Can you work these out from the model? Positions are in its coordinate system, mm. Face numbers are marked on the shaded views. A direction names the side the tool comes from. Give positions to 0.01 mm unless a question says otherwise; leave off trailing zeros. Order: outer loops, then holes, each group sorted by start corner. A loop starts at its lowest first (then second) coordinate and runs counter-clockwise, first axis right, second up. Notation, with made-up numbers: M -17,1.25 L 30,1.25 A6 cw 30,11.25 Z; hole C 47,21 d4. An arc over 180 degrees is marked long. Use one line per item in the form item = value. Start each with the question number.
1. I need wall thicknesses on L1, parallel to X at y = -2.45, z = -6.35 (3 decimals); L2, parallel to X at y = 29.5, z = 77 (3 decimals); L3, parallel to Z at x = 4, y = 66 (3 decimals). Which ranges of each line are inside material? Lowest first, please.
2. Will these pins go through, and if not, where does the flat tip stop? P1, Ø0.7, axis at y = 1, z = 3, coming from the +X side; P2, Ø7, axis at x = 153, z = 2, coming from the -Y side; P3, Ø1, axis at y = 35, z = 77, coming from the -X side (3 decimals); P4, Ø4, axis at x = 161.925, z = 44.45, coming from the -Y side (3 decimals).
3. I want a section at B-B, the plane z = 27. List the corners of the cut face in (x, y) for me (3 decimals), and give its area (3 significant figures).
4. We'd pull the mould along X, two halves only. Please class the marked faces 1, 2, 3 and 4: +X half, -X half, draft (parallel to the pull), parting line (faces both ways), or undercut.
5. I want a section at D-D, the plane x = 68. List the corners of the cut face in (y, z) for me (3 decimals), and give its area (3 significant figures).
6. I want a section at A-A, the plane z = 50.8. List the corners of the cut face in (x, y) for me (3 decimals), and give its area (3 significant figures).
7. I want a section at C-C, the plane y = 60.5. List the corners of the cut face in (x, z) for me (3 decimals).
8. For the marked faces 5 and 6, which set-ups out of +Z, -Z, +X, -X, +Y, -Y let a thin tool reach every point of the face, with its end or its side?
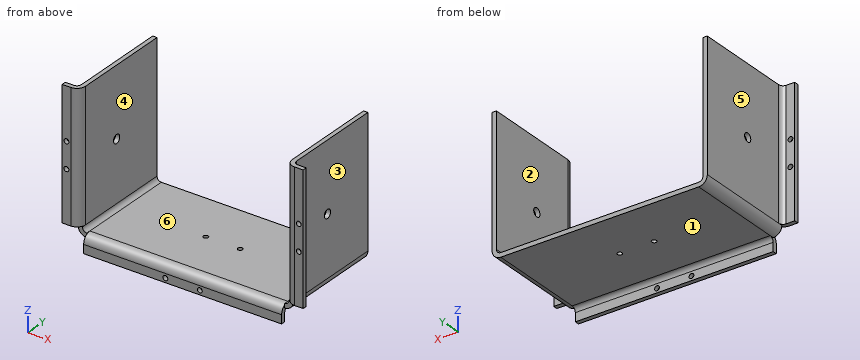
```python
from build123d import *

# Parameters (mm, degrees)
SKETCH1_W                    = 152.4
SKETCH1_H                    = 76.2
BOSS_EXTRUDE1_DEPTH          = 3.175
EDGE_FLANGE5_STRIP_W         = 19.05
EDGE_FLANGE5_STRIP_H         = 3.175
EDGE_FLANGE5_STRIP_CUT_DEPTH = 76.2
EDGE_FLANGE5_DEPTH           = 76.2
EDGE_FLANGE6_STRIP_W         = 19.05
EDGE_FLANGE6_STRIP_H         = 3.175
EDGE_FLANGE6_STRIP_CUT_DEPTH = 76.2
EDGE_FLANGE6_DEPTH           = 76.2
EDGE_FLANGE7_STRIP_W         = 19.05
EDGE_FLANGE7_STRIP_H         = 3.175
EDGE_FLANGE7_STRIP_CUT_DEPTH = 146.05
EDGE_FLANGE7_DEPTH           = 146.05
EDGE_FLANGE8_STRIP_W         = 19.05
EDGE_FLANGE8_STRIP_H         = 3.175
EDGE_FLANGE8_STRIP_CUT_DEPTH = 95.25
EDGE_FLANGE8_DEPTH           = 95.25
EDGE_FLANGE9_STRIP_W         = 19.05
EDGE_FLANGE9_STRIP_H         = 3.175
EDGE_FLANGE9_STRIP_CUT_DEPTH = 95.25
EDGE_FLANGE9_DEPTH           = 95.25
CUT_EXTRUDE1_DEPTH           = 211.820956323
CUT_EXTRUDE1_DEPTH_BACK      = 211.820956323
SKETCH60_R                   = 3.175
CUT_EXTRUDE2_DEPTH           = 207.765399971
CUT_EXTRUDE2_DEPTH_BACK      = 207.765399971
SKETCH61_R                   = 1.778
CUT_EXTRUDE3_DEPTH           = 209.295487229
CUT_EXTRUDE3_DEPTH_BACK      = 209.295487229
SKETCH62_R                   = 1.778


# Sheet-metal steps are written as plain solids
with BuildPart() as part:
    # Sketch1 → Boss-Extrude1 (new body)
    with BuildSketch(Plane.XY):
        with Locations((76.2, 38.1)):
            Rectangle(SKETCH1_W, SKETCH1_H)
    extrude(amount=BOSS_EXTRUDE1_DEPTH)

    # Edge-Flange5 strip (across the edge) → Edge-Flange5 strip cut (cut)
    with BuildSketch(Plane(origin=(152.4, 0, 3.175), x_dir=(-1, 0, 0), z_dir=(0, 1, 0))):
        with Locations((-6.35, -1.5875)):
            Rectangle(EDGE_FLANGE5_STRIP_W, EDGE_FLANGE5_STRIP_H)
    extrude(amount=EDGE_FLANGE5_STRIP_CUT_DEPTH, mode=Mode.SUBTRACT)

    # Edge-Flange5 section (across the edge) → Edge-Flange5 (add)
    with BuildSketch(Plane(origin=(152.4, 0, 3.175), x_dir=(-1, 0, 0), z_dir=(0, 1, 0))):
        with BuildLine():
            Line((-3.175, 3.175), (-3.175, 98.425))
            Line((-3.175, 98.425), (0, 98.425))
            Line((0, 98.425), (0, 3.175))
            ThreePointArc((0, 3.175), (0.92993597, 0.92993597), (3.175, 0))
            Line((3.175, 0), (3.175, -3.175))
            ThreePointArc((3.175, -3.175), (-1.315128061, -1.315128061), (-3.175, 3.175))
        make_face()
    extrude(amount=EDGE_FLANGE5_DEPTH)

    # Edge-Flange6 strip (across the edge) → Edge-Flange6 strip cut (cut)
    with BuildSketch(Plane(origin=(0, 76.2, 3.175), x_dir=(1, 0, 0), z_dir=(0, -1, 0))):
        with Locations((-6.35, -1.5875)):
            Rectangle(EDGE_FLANGE6_STRIP_W, EDGE_FLANGE6_STRIP_H)
    extrude(amount=EDGE_FLANGE6_STRIP_CUT_DEPTH, mode=Mode.SUBTRACT)

    # Edge-Flange6 section (across the edge) → Edge-Flange6 (add)
    with BuildSketch(Plane(origin=(0, 76.2, 3.175), x_dir=(1, 0, 0), z_dir=(0, -1, 0))):
        with BuildLine():
            Line((-3.175, 3.175), (-3.175, 98.425))
            Line((-3.175, 98.425), (0, 98.425))
            Line((0, 98.425), (0, 3.175))
            ThreePointArc((0, 3.175), (0.92993597, 0.92993597), (3.175, 0))
            Line((3.175, 0), (3.175, -3.175))
            ThreePointArc((3.175, -3.175), (-1.315128061, -1.315128061), (-3.175, 3.175))
        make_face()
    extrude(amount=EDGE_FLANGE6_DEPTH)

    # Edge-Flange7 strip (across the edge) → Edge-Flange7 strip cut (cut)
    with BuildSketch(Plane(origin=(149.225, 0, 0), x_dir=(0, 1, 0), z_dir=(-1, 0, 0))):
        with Locations((-6.35, -1.5875)):
            Rectangle(EDGE_FLANGE7_STRIP_W, EDGE_FLANGE7_STRIP_H)
    extrude(amount=EDGE_FLANGE7_STRIP_CUT_DEPTH, mode=Mode.SUBTRACT)

    # Edge-Flange7 section (across the edge) → Edge-Flange7 (add)
    with BuildSketch(Plane(origin=(149.225, 0, 0), x_dir=(0, 1, 0), z_dir=(-1, 0, 0))):
        with BuildLine():
            Line((-3.175, 3.175), (-3.175, 9.525))
            Line((-3.175, 9.525), (0, 9.525))
            Line((0, 9.525), (0, 3.175))
            ThreePointArc((0, 3.175), (0.92993597, 0.92993597), (3.175, 0))
            Line((3.175, 0), (3.175, -3.175))
            ThreePointArc((3.175, -3.175), (-1.315128061, -1.315128061), (-3.175, 3.175))
        make_face()
    extrude(amount=EDGE_FLANGE7_DEPTH)

    # Edge-Flange8 strip (across the edge) → Edge-Flange8 strip cut (cut)
    with BuildSketch(Plane(origin=(155.575, 0, 101.6), x_dir=(0, 1, 0), z_dir=(0, 0, -1))):
        with Locations((-6.35, -1.5875)):
            Rectangle(EDGE_FLANGE8_STRIP_W, EDGE_FLANGE8_STRIP_H)
    extrude(amount=EDGE_FLANGE8_STRIP_CUT_DEPTH, mode=Mode.SUBTRACT)

    # Edge-Flange8 section (across the edge) → Edge-Flange8 (add)
    with BuildSketch(Plane(origin=(155.575, 0, 101.6), x_dir=(0, 1, 0), z_dir=(0, 0, -1))):
        with BuildLine():
            Line((-3.175, 3.175), (-3.175, 9.525))
            Line((-3.175, 9.525), (0, 9.525))
            Line((0, 9.525), (0, 3.175))
            ThreePointArc((0, 3.175), (0.92993597, 0.92993597), (3.175, 0))
            Line((3.175, 0), (3.175, -3.175))
            ThreePointArc((3.175, -3.175), (-1.315128061, -1.315128061), (-3.175, 3.175))
        make_face()
    extrude(amount=EDGE_FLANGE8_DEPTH)

    # Edge-Flange9 strip (across the edge) → Edge-Flange9 strip cut (cut)
    with BuildSketch(Plane(origin=(-3.175, 0, 6.35), x_dir=(0, 1, 0), z_dir=(0, 0, 1))):
        with Locations((-6.35, -1.5875)):
            Rectangle(EDGE_FLANGE9_STRIP_W, EDGE_FLANGE9_STRIP_H)
    extrude(amount=EDGE_FLANGE9_STRIP_CUT_DEPTH, mode=Mode.SUBTRACT)

    # Edge-Flange9 section (across the edge) → Edge-Flange9 (add)
    with BuildSketch(Plane(origin=(-3.175, 0, 6.35), x_dir=(0, 1, 0), z_dir=(0, 0, 1))):
        with BuildLine():
            Line((-3.175, 3.175), (-3.175, 9.525))
            Line((-3.175, 9.525), (0, 9.525))
            Line((0, 9.525), (0, 3.175))
            ThreePointArc((0, 3.175), (0.92993597, 0.92993597), (3.175, 0))
            Line((3.175, 0), (3.175, -3.175))
            ThreePointArc((3.175, -3.175), (-1.315128061, -1.315128061), (-3.175, 3.175))
        make_face()
    extrude(amount=EDGE_FLANGE9_DEPTH)

    # Sketch60 → Cut-Extrude1 (cut, two sides: drawn at the far end of the back side and taken through both)
    with BuildSketch(Plane(origin=(155.575, 0, 0), x_dir=(0, 0, -1), z_dir=(1, 0, 0)).offset(-CUT_EXTRUDE1_DEPTH_BACK)):
        with Locations(Location((-50.8, 34.925, 0), (0, 0, 180))):
            Circle(SKETCH60_R)
    extrude(amount=CUT_EXTRUDE1_DEPTH + CUT_EXTRUDE1_DEPTH_BACK, mode=Mode.SUBTRACT)

    # Sketch61 → Cut-Extrude2 (cut, two sides: drawn at the far end of the back side and taken through both)
    with BuildSketch(Plane.XY.offset(3.175).offset(-CUT_EXTRUDE2_DEPTH_BACK)):
        with Locations((88.9, 38.1)):
            Circle(SKETCH61_R)
        with Locations((63.5, 38.1)):
            Circle(SKETCH61_R)
    extrude(amount=CUT_EXTRUDE2_DEPTH + CUT_EXTRUDE2_DEPTH_BACK, mode=Mode.SUBTRACT)

    # Sketch62 → Cut-Extrude3 (cut, two sides: drawn at the far end of the back side and taken through both)
    with BuildSketch(Plane(origin=(0, 0, 0), x_dir=(1, 0, 0), z_dir=(0, 1, 0)).offset(-CUT_EXTRUDE3_DEPTH_BACK)):
        with Locations(Location((63.5, 6.35, 0), (0, 0, 270))):
            Circle(SKETCH62_R)
        with Locations(Location((-9.525, -44.45, 0), (0, 0, 270))):
            Circle(SKETCH62_R)
        with Locations(Location((-9.525, -63.5, 0), (0, 0, 270))):
            Circle(SKETCH62_R)
        with Locations(Location((161.925, -63.5, 0), (0, 0, 90))):
            Circle(SKETCH62_R)
        with Locations(Location((161.925, -44.45, 0), (0, 0, 90))):
            Circle(SKETCH62_R)
        with Locations(Location((88.9, 6.35, 0), (0, 0, 90))):
            Circle(SKETCH62_R)
    extrude(amount=CUT_EXTRUDE3_DEPTH + CUT_EXTRUDE3_DEPTH_BACK, mode=Mode.SUBTRACT)


solid = part.part
```
Check result:
q1.L1 = 3.175 to 61.722, 65.278 to 87.122, 90.678 to 149.225
q1.L2 = -3.175 to 0, 152.4 to 155.575
q1.L3 = 0 to 3.175
q2.P1 = 154.82
q2.P2 = 0
q2.P3 = -3.175
q2.P4 = -3.175
q3.outline = M -12.7,-3.175 L -6.35,-3.175 A6.35 ccw 0,3.175 L 0,76.2 L -3.175,76.2 L -3.175,3.175 A3.175 cw -6.35,0 L -12.7,0 Z; M 152.4,3.175 A6.35 ccw 158.75,-3.175 L 165.1,-3.175 L 165.1,0 L 158.75,0 A3.175 cw 155.575,3.175 L 155.575,76.2 L 152.4,76.2 Z
q3.area = 552 mm2
q4.face_1 = draft
q4.face_2 = undercut
q4.face_3 = +X half
q4.face_4 = undercut
q5.outline = M -3.175,-9.525 L 0,-9.525 L 0,-3.175 A3.175 cw 3.175,0 L 76.2,0 L 76.2,3.175 L 3.175,3.175 A6.35 ccw -3.175,-3.175 Z
q5.area = 276 mm2
q6.outline = M -12.7,-3.175 L -6.35,-3.175 A6.35 ccw 0,3.175 L 0,31.75 L -3.175,31.75 L -3.175,3.175 A3.175 cw -6.35,0 L -12.7,0 Z; M -3.175,38.1 L 0,38.1 L 0,76.2 L -3.175,76.2 Z; M 152.4,3.175 A6.35 ccw 158.75,-3.175 L 165.1,-3.175 L 165.1,0 L 158.75,0 A3.175 cw 155.575,3.175 L 155.575,31.75 L 152.4,31.75 Z; M 152.4,38.1 L 155.575,38.1 L 155.575,76.2 L 152.4,76.2 Z
q6.area = 511 mm2
q7.outline = M -3.175,6.35 A6.35 ccw 3.175,0 L 149.225,0 A6.35 ccw 155.575,6.35 L 155.575,101.6 L 152.4,101.6 L 152.4,6.35 A3.175 cw 149.225,3.175 L 3.175,3.175 A3.175 cw 0,6.35 L 0,101.6 L -3.175,101.6 Z
q8.face_5 = +Z, -Z, -X, +Y
q8.face_6 = +Z, +Y, -Y
